from build123d import *

# Parameters (mm, degrees)
SKETCH_1_W          = 55
SKETCH_1_H          = 55
EXTRUDE_1_DEPTH     = 50
CUT_EXTRUDE_1_DEPTH = 38
EXTRUDE_2_REACH     = 81.254
EXTRUDE_START       = -5
EXTRUDE_3_DEPTH     = 10
EXTRUDE_START_2     = -8
EXTRUDE_4_DEPTH     = 10
SKETCH_6_W          = 10
SKETCH_6_H          = 8
CUT_EXTRUDE_2_DEPTH = 15


with BuildPart() as part:
    # Эскиз1 → Бобышка-Вытянуть1 (new body)
    with BuildSketch(Plane.XY):
        Rectangle(SKETCH_1_W, SKETCH_1_H)
    extrude(amount=EXTRUDE_1_DEPTH)

    # Эскиз2 → Вырез-Вытянуть1 (cut)
    with BuildSketch(Plane.XZ.offset(27.5)):
        Polygon((-27.5, 15), (7.5, 15), (7.5, 30), (27.5, 50), (-27.5, 50), align=None)
    extrude(amount=-CUT_EXTRUDE_1_DEPTH, mode=Mode.SUBTRACT)

    # Бобышка-Вытянуть2: up to this face of the body (flat: up to its plane)
    extrude_2_end = Plane(part.part.faces().sort_by_distance((27.5, 0, 25))[0])
    # Эскиз3 → Бобышка-Вытянуть2 (add, up to the picked face)
    with BuildSketch(Plane.ZY.offset(27.5), mode=Mode.PRIVATE) as extrude_2_sk1:
        Polygon((50, 10.5), (15, -13.5), (15, 10.5), align=None)
    extrude_2_tool1 = split(extrude(extrude_2_sk1.sketch, amount=-EXTRUDE_2_REACH, mode=Mode.PRIVATE), bisect_by=extrude_2_end, keep=Keep.BOTH, mode=Mode.PRIVATE)
    add(extrude_2_tool1.solids().sort_by(Axis((-27.5, 2.5, 26.666667), (1, 0, 0)))[0])

    # Эскиз4 → Бобышка-Вытянуть3 (add)
    with BuildSketch(Plane.ZY.offset(27.5).offset(EXTRUDE_START)):
        Polygon((32.5, -1.5), (32.5, -13.5), (15, -13.5), align=None)
    extrude(amount=-EXTRUDE_3_DEPTH)

    # Эскиз5 → Бобышка-Вытянуть4 (add)
    with BuildSketch(Plane.XZ.offset(27.5).offset(EXTRUDE_START_2)):
        with BuildLine():
            Line((27.5, 50), (7.5, 30))
            ThreePointArc((7.5, 30), (13.357864376, 44.142135624), (27.5, 50))
        make_face()
    extrude(amount=-EXTRUDE_4_DEPTH)

    # Эскиз6 → Вырез-Вытянуть2 (cut)
    with BuildSketch(Plane.ZY.offset(27.5)):
        with Locations((5, 23.5)):
            Rectangle(SKETCH_6_W, SKETCH_6_H)
    extrude(amount=-CUT_EXTRUDE_2_DEPTH, mode=Mode.SUBTRACT)


solid = part.part
Could you check a few things on this model? Use its own coordinates, in mm. A direction names the side the tool comes from. Round coordinates to 2 decimals unless told otherwise and drop trailing zeros. Order: outer loops, then holes, each group sorted by start corner. A loop starts at its lowest first (then second) coordinate and runs counter-clockwise, first axis right, second up.
(1) Imagine slicing it at A-A (z = 34). Write out the boundary of the cut face in (x, y).
Response values:
outline: (-27.5, -0.47) - (11.5, -0.47) - (11.5, -9.5) - (7.9, -9.5) - (7.9, -19.5) - (11.5, -19.5) - (11.5, -27.5) - (27.5, -27.5) - (27.5, 27.5) - (-27.5, 27.5) - close
(2) I'm going to push flat-ended pins straight in: pin 1 (1.5 mm diameter, centred on x = 18.5, y = -17, fed in from +Z); pin 2 (8 mm diameter, centred on x = -18.5, z = 25.5, fed in from -Y); pin 3 (6.5 mm diameter, centred on y = 24, z = 3.5, fed in from -X). Where does each tip first touch, or does it pass through?
Response values:
pin 1: stops at z = 48.22
pin 2: stops at y = -13.5
pin 3: stops at x = -12.5
(3) Which directions (+Z, -Z, +X, -X, +Y, -Y) give clear straight access to the entire face, cutting with the end or side of a thin tool? Please do faces 1 (the flat face through (-10, -21, 15)), 2 (the flat face through (0, 27.5, 25)), 3 (the flat face through (-20, 19.5, 5)).
Response values:
face 1: +Z, -X, -Y
face 2: +Z, -Z, +X, -X, +Y
face 3: -Z, -X, +Y
(4) If we mould it in two halves opening along X, with no side actions, what happens to faces 4 (the flat face through (6, -27.5, 14)), 5 (the flat face through (-12.5, 24, 5)), 6 (the flat face through (7.5, -18, 22)), 7 (the flat face through (-12.5, -10, 28))? For each: released by +X, released by -X, zero draft, split by the parting line, or undercut.
Response values:
face 4: zero draft
face 5: released by -X
face 6: undercut
face 7: undercut
(5) Imagine slicing it at C-C (y = -18.5). Write out the boundary of the cut face in (x, z).
Response values:
outline: (-27.5, 0) - (27.5, 0) - (27.5, 50) arc R20 ccw to (7.5, 30) - (7.5, 15) - (-27.5, 15) - close
(6) Imagine slicing it at B-B (x = -10). Write out the boundary of the cut face in (y, z).
Response values:
outline: (-27.5, 0) - (27.5, 0) - (27.5, 50) - (10.5, 50) - (-13.5, 15) - (-27.5, 15) - close
(7) Imagine slicing it at D-D (z = 46). Write out the boundary of the cut face in (x, y), plus the area to 3 significant figures.
Response values:
outline: (-27.5, 7.76) - (23.5, 7.76) - (23.5, -9.5) - (15.5, -9.5) - (15.5, -19.5) - (23.5, -19.5) - (23.5, -27.5) - (27.5, -27.5) - (27.5, 27.5) - (-27.5, 27.5) - close
area: 1,310 mm2
(8) Please list where these lines run through material, in increasing order: line 1 along Z through (x, y) = (-0.5, -23.5); line 2 along Y through (x, z) = (-17, 25); line 3 along Y through (x, z) = (-15.5, 5.5).
Response values:
line 1: z = 0 to 15
line 2: y = -13.5 to 27.5
line 3: y = -27.5 to 19.5
